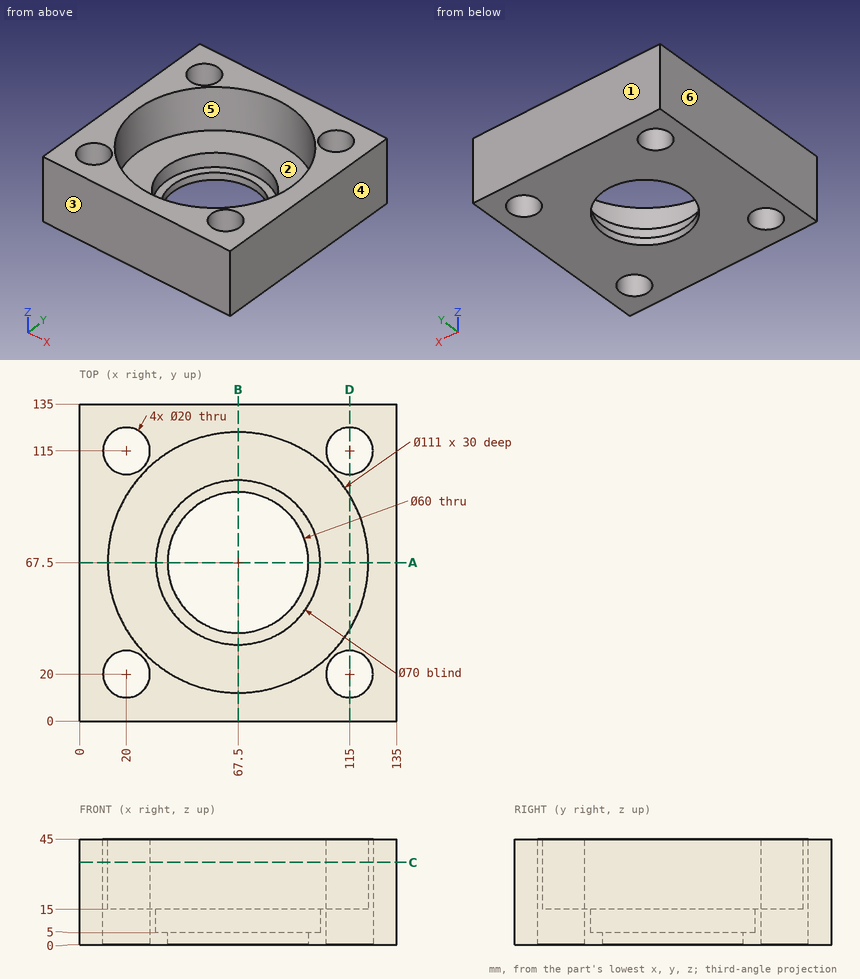
Source: three-view drawing plus pictorial views. Frame: mm from the lowest corner of the part. A direction names the side the tool comes from. Coordinates: 2 decimals unless noted, no trailing zeros. Loops run counter-clockwise (first coordinate to the right, second up) from the corner with the lowest first, then second, coordinate; pieces in that order, holes last. Notation, with made-up numbers: (22, 83.5) -> (68, 83.5) arc R10 cw to (68, 93.5) -> close; hole circle Ø4 at (21.25, 24.25). An arc over 180 degrees is marked (long way). One line per item, written item: value.
(1) Pin query (flat end, axial travel): pin 1 Ø12 at (x, z) = (45, 33) entering from -Y. Return the tip coordinate at first contact, or that it passes through.
Answer below:
pin 1: stops at y = 0
(2) Cut plane C-C (z = 35). Output: boundary loops of the cut face in (x, y).
Answer below:
outline: (0, 0) -> (135, 0) -> (135, 135) -> (0, 135) -> close; hole circle Ø20 at (20, 20); hole circle Ø20 at (20, 115); hole circle Ø111 at (67.5, 67.5); hole circle Ø20 at (115, 20); hole circle Ø20 at (115, 115)
(3) Ray query, line 1 along Y through (x, z) = (20, 24); line 2 along Y through (x, z) = (112.5, 42); line 3 along X through (y, z) = (66, 39.5). Return the intervals inside material, ascending.
Answer below:
line 1: y = 0 to 10, 30 to 38.79, 96.21 to 105, 125 to 135
line 2: y = 0 to 10.32, 29.68 to 35.02, 99.98 to 105.32, 124.68 to 135
line 3: x = 0 to 12.02, 122.98 to 135
(4) Cut plane A-A (y = 67.5). Output: boundary loops of the cut face in (x, z).
Answer below:
outline: (0, 0) -> (37.5, 0) -> (37.5, 5) -> (32.5, 5) -> (32.5, 15) -> (12, 15) -> (12, 45) -> (0, 45) -> close; (97.5, 0) -> (135, 0) -> (135, 45) -> (123, 45) -> (123, 15) -> (102.5, 15) -> (102.5, 5) -> (97.5, 5) -> close
(5) Cut plane D-D (x = 115). Output: boundary loops of the cut face in (y, z).
Answer below:
outline: (0, 0) -> (10, 0) -> (10, 45) -> (0, 45) -> close; (30, 0) -> (105, 0) -> (105, 45) -> (96.21, 45) -> (96.21, 15) -> (38.79, 15) -> (38.79, 45) -> (30, 45) -> close; (125, 0) -> (135, 0) -> (135, 45) -> (125, 45) -> close
(6) Set-up query: the marked faces 1 and 2. Return all of +Z, -Z, +X, -X, +Y, -Y with unobstructed straight access to the full face (end or side cutting, diameter ignored); none if empty.
Answer below:
face 1: +Z, -Z, +X, -X, +Y
face 2: +Z
(7) Draft query along X for the marked faces 3, 4, 5 and 6. Return one class per face: pulls with the +X half, pulls with the -X half, needs draft (parallel to the pull), parting line crosses it, or undercut.
Answer below:
face 3: needs draft
face 4: pulls with the +X half
face 5: undercut
face 6: pulls with the -X half
